Check sheet for the modelled part. Datum: model origin and axes. Units: mm. Face numbers are marked on the shaded views. A direction names the side the tool comes from. Give positions to 0.01 mm unless a question says otherwise; leave off trailing zeros. Order: outer loops, then holes, each group sorted by start corner. A loop starts at its lowest first (then second) coordinate and runs counter-clockwise, first axis right, second up.
Item 1: Gauge pin test, flat ends, axial feed: P1, Ø2.5, axis at x = 0.5, z = -51, coming from the -Y side; P2, Ø2, axis at y = -3, z = -49, coming from the +X side; P3, Ø1.8, axis at x = 1.5, y = 1, coming from the -Z side. Record the tip position at first contact, or that the pin passes through.
Item 2: Sectioned sample at D-D on x = 5.25. Record the boundary of the cut face in (y, z), and give its area (3 significant figures).
Item 3: Material ranges on line 1 along Z through (x, y) = (-4, 2.5); line 2 along Z through (x, y) = (-6.5, -1.25); line 3 along Y through (x, z) = (-1, -52), recorded low to high.
Item 4: Sectioned sample at A-A on y = 5.25. Record the boundary of the cut face in (x, z), and give its area (3 significant figures).
Item 5: Access from +Z, -Z, +X, -X, +Y, -Y to the whole of each face (thin tool, end or side, straight path). Record for the marked faces 4 and 5.
Item 6: Sectioned sample at C-C on z = 15. Record the boundary of the cut face in (x, y), and give its area (3 significant figures).
Item 7: Sectioned sample at B-B on x = 0. Record the boundary of the cut face in (y, z).
Item 8: Release check for a two-part mould opening along Z. For the marked faces 1, 2 and 3 record: released by +Z, released by -Z, zero draft, split by the parting line, or undercut.
from build123d import *

# Parameters (mm, degrees)
BOSS_EXTRUDE1_DEPTH = 27
SKETCH2_R           = 4.5
BOSS_EXTRUDE2_DEPTH = 61
CUT_EXTRUDE1_DEPTH  = 14
SKETCH4_R           = 6
BOSS_EXTRUDE3_DEPTH = 33


with BuildPart() as part:
    # Sketch1 → Boss-Extrude1 (new body)
    with BuildSketch(Plane.XY):
        Polygon((3.666174209, -6.35), (7.332348419, 0), (3.666174209, 6.35), (-3.666174209, 6.35), (-7.332348419, 0), (-3.666174209, -6.35), align=None)
    extrude(amount=BOSS_EXTRUDE1_DEPTH)

    # Sketch2 → Boss-Extrude2 (add)
    with BuildSketch(Plane(origin=(0, 0, 0), x_dir=(-1, 0, 0), z_dir=(0, 0, -1))):
        with Locations(Location((0, 0, 0), (0, 0, 180))):
            Circle(SKETCH2_R)
    extrude(amount=BOSS_EXTRUDE2_DEPTH)

    # Sketch3 → Cut-Extrude1 (cut)
    with BuildSketch(Plane(origin=(0, 0, -61), x_dir=(-1, 0, 0), z_dir=(0, 0, -1))):
        with BuildLine():
            Line((-2.645751311, 3), (2.645751311, 3))
            ThreePointArc((2.645751311, 3), (4, 0), (2.645751311, -3))
            Line((2.645751311, -3), (-2.645751311, -3))
            ThreePointArc((-2.645751311, -3), (-4, 0), (-2.645751311, 3))
        make_face()
    extrude(amount=-CUT_EXTRUDE1_DEPTH, mode=Mode.SUBTRACT)

    # Sketch4 → Boss-Extrude3 (add)
    with BuildSketch(Plane(origin=(0, 0, -61), x_dir=(-1, 0, 0), z_dir=(0, 0, -1))):
        Circle(SKETCH4_R)
        with BuildLine():
            Line((-2.645751311, -3), (2.645751311, -3))
            ThreePointArc((2.645751311, -3), (4, 0), (2.645751311, 3))
            Line((2.645751311, 3), (-2.645751311, 3))
            ThreePointArc((-2.645751311, 3), (-4, 0), (-2.645751311, -3))
        make_face(mode=Mode.SUBTRACT)
    extrude(amount=-BOSS_EXTRUDE3_DEPTH)


solid = part.part
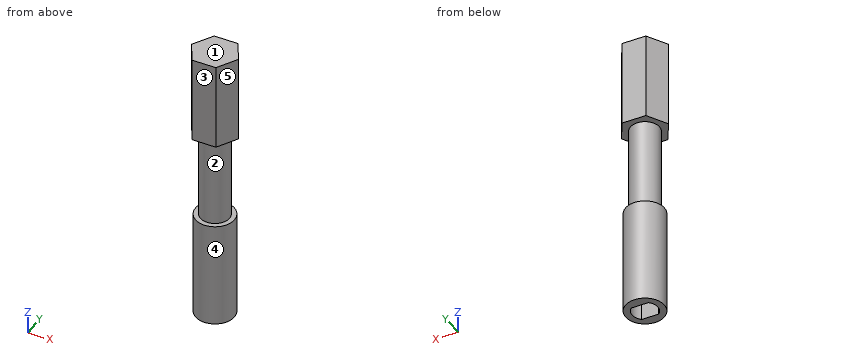
Report:
1. P1: stops at y = -6
1. P2: stops at x = 5.66
1. P3: stops at z = -47
2. outline: (-3.61, 0) - (3.61, 0) - (3.61, 27) - (-3.61, 27) - close; (-2.9, -61) - (2.9, -61) - (2.9, -28) - (-2.9, -28) - close
2. area: 386 mm2
3. line 1: z = -61 to -28, 0 to 27
3. line 2: z = 0 to 27
3. line 3: y = -5.92 to -3, 3 to 5.92
4. outline: (-4.3, 0) - (4.3, 0) - (4.3, 27) - (-4.3, 27) - close; (-2.9, -61) - (2.9, -61) - (2.9, -28) - (-2.9, -28) - close
4. area: 424 mm2
5. face 4: -Z
5. face 5: +Z, -Z, +X, -Y
6. outline: (-7.33, 0) - (-3.67, -6.35) - (3.67, -6.35) - (7.33, 0) - (3.67, 6.35) - (-3.67, 6.35) - close
6. area: 140 mm2
7. outline: (-6.35, 0) - (-4.5, 0) - (-4.5, -28) - (-6, -28) - (-6, -61) - (-3, -61) - (-3, -47) - (3, -47) - (3, -61) - (6, -61) - (6, -28) - (4.5, -28) - (4.5, 0) - (6.35, 0) - (6.35, 27) - (-6.35, 27) - close
8. face 1: released by +Z
8. face 2: undercut
8. face 3: zero draft
